Build history of the part. All positions in model axes, mm. A direction names the side the tool comes from. Give positions to 0.01 mm unless a question says otherwise; leave off trailing zeros. Order: outer loops, then holes, each group sorted by start corner. A loop starts at its lowest first (then second) coordinate and runs counter-clockwise, first axis right, second up. Notation, with made-up numbers: (-11.5, -14.75) -> (6.5, -14.75) arc R25 cw to (6.5, 22.25) -> close; hole circle Ø2 at (69.25, 33.25). An arc over 180 degrees is marked (long way). One line per item, written item: value. Start each with the question number.
(1) Two-plate mould, pull along X, no slides. Class faces 1 (the cylindrical face through (29.062, 87.551, 68.63)), 2 (the flat face through (3.48, 114.53, -1.33)), 3 (the cylindrical face through (28.115, 111.263, 44.917)), 4 (the flat face through (-21.93, 96.807, 46.665)): +X half, -X half, draft (parallel to the pull), parting line (faces both ways), or undercut.
(2) Pin check, flat tips, straight feed: pin 1 (2 mm diameter, centred on x = -30, z = -10, fed in from -Y); pin 2 (3 mm diameter, centred on x = -11.5, z = 65, fed in from -Y) (3 decimals); pin 3 (5 mm diameter, centred on y = 64.5, z = 21, fed in from +X); pin 4 (4.5 mm diameter, centred on x = 8.41, y = 69.57, fed in from -Z). Stop position of each tip, or through.
(3) Saw through at D-D on x = -3. Give the cut face in (y, z), plus the area to 3 significant figures.
(4) Probe line 1 (Y direction, x = 8, z = -25); line 2 (Z direction, x = -25.5, y = 103.5); line 3 (Z direction, x = 26.5, y = 53). List the from-to ranges inside material, lowest first.
(5) Saw through at C-C on z = 59. Give the cut face in (x, y), plus the area to 3 significant figures.
(6) Which spindle directions (+Z, -Z, +X, -X, +Y, -Y) get a long thin tool onto all of the face, cutting with end or side? Do faces 5 (the flat face through (-27, 78, 23)), 6 (the flat face through (37, 113, 40)), 7 (the flat face through (-29, 87.896, -9)). Say none if no direction does.
(7) Saw through at B-B on y = 60. Give the cut face in (x, z).
(8) Saw through at A-A on x = 8.41. Give the cut face in (y, z), plus the area to 3 significant figures.
```python
from build123d import *

# Parameters (mm, degrees)
BOSS_EXTRUDE1_DEPTH      = 37
BOSS_EXTRUDE1_DEPTH_BACK = 27
SKETCH2_R                = 2
CUT_EXTRUDE1_DEPTH       = 179.149132383
BOSS_EXTRUDE2_DEPTH      = 4
CHAMFER1_SIZE            = 15
SKETCH4_R                = 3
CUT_EXTRUDE7_DEPTH       = 20
CHAMFER2_SIZE            = 10


with BuildPart() as part:
    # Sketch1 → Boss-Extrude1 (new, two sides: drawn at the far end of the back side and taken through both)
    with BuildSketch(Plane(origin=(0, 0, 0), x_dir=(0, 0, -1), z_dir=(1, 0, 0)).offset(-BOSS_EXTRUDE1_DEPTH_BACK)):
        Polygon((22.304433561, 10.566780625), (22.304433561, 87.896140672), (-20.12197331, 130.322547544), (-77.397622586, 73.046898267), (-83.054476835, 78.703752517), (-22.950400434, 138.807828918), (26.304433561, 89.552994922), (26.304433561, 10.566780625), align=None)
    extrude(amount=BOSS_EXTRUDE1_DEPTH + BOSS_EXTRUDE1_DEPTH_BACK)

    # Sketch2 → Cut-Extrude1 (cut, through all)
    with BuildSketch(Plane.XY.offset(-22.304433561)):
        with Locations((8.41, 69.566780625)):
            Circle(SKETCH2_R)
        with Locations((26.41, 47.066780625)):
            Circle(SKETCH2_R)
        with Locations((8.41, 24.566780625)):
            Circle(SKETCH2_R)
        with Locations((-9.59, 47.066780625)):
            Circle(SKETCH2_R)
    extrude(amount=-CUT_EXTRUDE1_DEPTH, mode=Mode.SUBTRACT)

    # Sketch12 → Boss-Extrude2 (add)
    with BuildSketch(Plane.ZY.offset(27)):
        Polygon((-22.304433561, 10.566780625), (-19.7923121, 10.566780625), (77.397622586, 73.046898267), (20.12197331, 130.322547544), (-22.304433561, 87.896140672), (5.695566439, 87.896140672), (5.695566439, 32.896140672), (-22.304433561, 32.896140672), align=None)
        Polygon((-26.304433561, 89.552994922), (-26.304433561, 10.566780625), (-22.304433561, 10.566780625), (-22.304433561, 87.896140672), (20.12197331, 130.322547544), (77.397622586, 73.046898267), (83.054476835, 78.703752517), (22.950400434, 138.807828918), align=None)
    extrude(amount=BOSS_EXTRUDE2_DEPTH)

    # Chamfer1
    chamfer1_edges = [part.edges().sort_by_distance(p)[0] for p in [
        (5, 130.322547544, 20.12197331),
    ]]
    chamfer(chamfer1_edges, length=CHAMFER1_SIZE)

    # Sketch4 → Cut-Extrude7 (cut)
    with BuildSketch(Plane(origin=(0, 204.733202838, -42.974973485), x_dir=(1, 0, 0), z_dir=(0, -0.7071067811865472, -0.7071067811865478))):
        with Locations(Location((-9.26766953, 126.031352928, 0), (0, 0, 270))):
            Circle(SKETCH4_R)
        with Locations(Location((-9.26766953, 161.386691988, 0), (0, 0, 270))):
            Circle(SKETCH4_R)
        with Locations(Location((26.08766953, 161.386691988, 0), (0, 0, 270))):
            Circle(SKETCH4_R)
        with Locations(Location((26.08766953, 126.031352928, 0), (0, 0, 270))):
            Circle(SKETCH4_R)
    extrude(amount=CUT_EXTRUDE7_DEPTH, mode=Mode.SUBTRACT)

    # Chamfer2
    chamfer2_edges = [part.edges().sort_by_distance(p)[0] for p in [
        (-27, 96.381422047, 54.063098807),
    ]]
    chamfer(chamfer2_edges, length=CHAMFER2_SIZE)


solid = part.part
```
Results below:
1. face 1: undercut
1. face 2: draft
1. face 3: undercut
1. face 4: +X half
2. pin 1: stops at y = 16.22
2. pin 2: stops at y = 84.015
2. pin 3: stops at x = -27
2. pin 4: stops at z = -26.3
3. outline: (10.57, -26.3) -> (89.55, -26.3) -> (138.81, 22.95) -> (78.7, 83.05) -> (73.05, 77.4) -> (119.72, 30.73) -> (119.72, 9.52) -> (87.9, -22.3) -> (10.57, -22.3) -> close
3. area: 1,350 mm²
4. line 1: y = 10.57 to 22.61, 26.52 to 67.61, 71.52 to 90.86
4. line 2: z = -12.36 to -6.7, 34.92 to 58.26
4. line 3: z = -26.3 to -22.3
5. outline: (-31, 61.22) -> (-27, 61.22) -> (-27, 77.3) -> (-17, 91.44) -> (37, 91.44) -> (37, 102.76) -> (-31, 102.76) -> close
5. area: 961 mm²
6. face 5: +X, -Y
6. face 6: +Z, -Z, +X, +Y, -Y
6. face 7: +X, -X
7. outline: (-31, -26.3) -> (37, -26.3) -> (37, -22.3) -> (-31, -22.3) -> close; (-31, 5.7) -> (-27, 5.7) -> (-27, 57.1) -> (-31, 57.1) -> close
8. outline: (10.57, -26.3) -> (22.57, -26.3) -> (22.57, -22.3) -> (10.57, -22.3) -> close; (26.57, -26.3) -> (67.57, -26.3) -> (67.57, -22.3) -> (26.57, -22.3) -> close; (71.57, -26.3) -> (89.55, -26.3) -> (138.81, 22.95) -> (78.7, 83.05) -> (73.05, 77.4) -> (119.72, 30.73) -> (119.72, 9.52) -> (87.9, -22.3) -> (71.57, -22.3) -> close
8. area: 1,320 mm²
